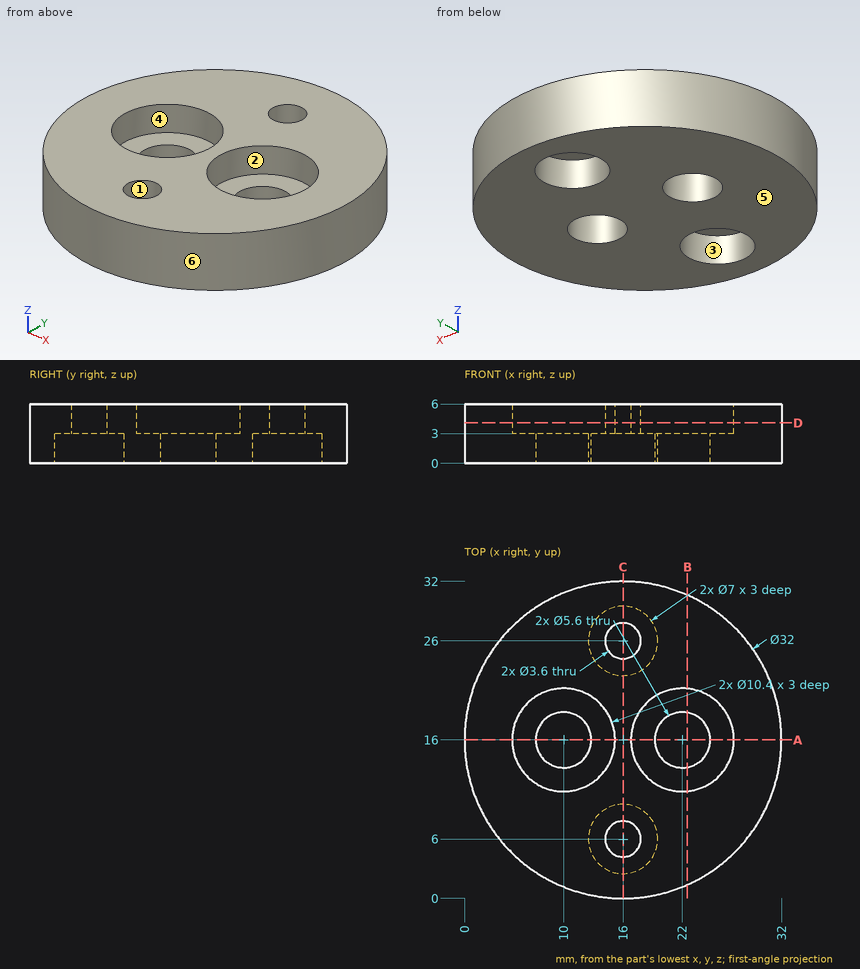
Geometry: see drawing. Coordinates: mm, zero at the bounding-box minimum. A direction names the side the tool comes from. Give positions to 0.01 mm unless a question says otherwise; leave off trailing zeros. Order: outer loops, then holes, each group sorted by start corner. A loop starts at its lowest first (then second) coordinate and runs counter-clockwise, first axis right, second up. Notation, with made-up numbers: (43, 26.5) -> (73, 26.5) arc R20 cw to (73, 51.5) -> close; hole circle Ø8 at (85.25, 81). An arc over 180 degrees is marked (long way). Write each question's results on one line, items separated by ' | '. Start each with the question number.
1) Draft query along Y for the marked faces 4, 5 and 6. Return one class per face: pulls with the +Y half, pulls with the -Y half, needs draft (parallel to the pull), parting line crosses it, or undercut.
2) Section C-C (x = 16). Return loops of the section in (y, z).
3) Set-up query: the marked faces 1, 2 and 3. Return all of +Z, -Z, +X, -X, +Y, -Y with unobstructed straight access to the full face (end or side cutting, diameter ignored); none if empty.
4) Section D-D (z = 4.1). Return loops of the section in (x, y), then the cut area to 3 significant figures.
5) First-contact query: pin 1 (4.5 mm diameter, centred on x = 16, y = 26, fed in from -Z); pin 2 (6 mm diameter, centred on x = 22, y = 16, fed in from -Z); pin 3 (1 mm diameter, centred on y = 19, z = 1, fed in from +X); pin 4 (1.5 mm diameter, centred on x = 28.5, z = 1.5, fed in from +Y). Flat tips, straight axial feed; report the tip coordinate or a pass-through.
6) Section A-A (y = 16). Return loops of the section in (x, z).
7) Section B-B (x = 22.5). Return loops of the section in (y, z) (3 decimals).
8) Line query: line 1 (X direction, y = 15.5, z = 2.35) (3 decimals); line 2 (Y direction, x = 12, z = 2.5); line 3 (Y direction, x = 23.5, z = 2.85). Output: solid intervals per line, ascending. Write a range as from..to.
Calculated:
1) face 4: undercut | face 5: needs draft | face 6: parting line crosses it
2) outline: (0, 0) -> (2.5, 0) -> (2.5, 3) -> (4.2, 3) -> (4.2, 6) -> (0, 6) -> close; (7.8, 3) -> (9.5, 3) -> (9.5, 0) -> (22.5, 0) -> (22.5, 3) -> (24.2, 3) -> (24.2, 6) -> (7.8, 6) -> close; (27.8, 3) -> (29.5, 3) -> (29.5, 0) -> (32, 0) -> (32, 6) -> (27.8, 6) -> close
3) face 1: +Z, -Z | face 2: +Z | face 3: -Z
4) outline: circle Ø32 at (16, 16); hole circle Ø10.4 at (10, 16); hole circle Ø3.6 at (16, 6); hole circle Ø3.6 at (16, 26); hole circle Ø10.4 at (22, 16) | area: 614 mm2
5) pin 1: z = 3 | pin 2: z = 0 | pin 3: x = 31.8 | pin 4: y = 26.86
6) outline: (0, 0) -> (7.2, 0) -> (7.2, 3) -> (4.8, 3) -> (4.8, 6) -> (0, 6) -> close; (12.8, 0) -> (19.2, 0) -> (19.2, 3) -> (16.8, 3) -> (16.8, 6) -> (15.2, 6) -> (15.2, 3) -> (12.8, 3) -> close; (24.8, 0) -> (32, 0) -> (32, 6) -> (27.2, 6) -> (27.2, 3) -> (24.8, 3) -> close
7) outline: (1.38, 0) -> (13.245, 0) -> (13.245, 3) -> (10.824, 3) -> (10.824, 6) -> (1.38, 6) -> close; (18.755, 0) -> (30.62, 0) -> (30.62, 6) -> (21.176, 6) -> (21.176, 3) -> (18.755, 3) -> close
8) line 1: 0.008..7.245, 12.755..19.245, 24.755..31.992 | line 2: 0.51..14.04, 17.96..31.49 | line 3: 1.87..13.64, 18.36..30.13
